from build123d import *

# Parameters (mm, degrees)
SKETCH_1_R      = 3.5
SKETCH_1_W      = 9.2
SKETCH_1_H      = 9.2
EXTRUDE_3_DEPTH = 100


with BuildPart() as part:
    # 草图1 → 凸台-拉伸3 (new body)
    with BuildSketch(Plane.XY):
        with BuildLine():
            Line((-27, 17), (-27, 9.314213562))
            Line((-27, 9.314213562), (-26.241421356, 9.314213562))
            ThreePointArc((-26.241421356, 9.314213562), (-26.149033403, 9.252481906), (-26.170710678, 9.143502884))
            Line((-26.170710678, 9.143502884), (-26.707106781, 8.607106781))
            Line((-26.707106781, 8.607106781), (-22.086856928, 3.986856928))
            ThreePointArc((-22.086856928, 3.986856928), (-20, 4.5), (-17.913143072, 3.986856928))
            Line((-17.913143072, 3.986856928), (-13.292893219, 8.607106781))
            Line((-13.292893219, 8.607106781), (-13.829289322, 9.143502884))
            ThreePointArc((-13.829289322, 9.143502884), (-13.850966597, 9.252481906), (-13.758578644, 9.314213562))
            Line((-13.758578644, 9.314213562), (-13, 9.314213562))
            Line((-13, 9.314213562), (-13, 17))
            Line((-13, 17), (-14.95, 17))
            Line((-14.95, 17), (-14.95, 18.5))
            ThreePointArc((-14.95, 18.5), (-14.510660172, 19.560660172), (-13.45, 20))
            Line((-13.45, 20), (13.45, 20))
            ThreePointArc((13.45, 20), (14.510660172, 19.560660172), (14.95, 18.5))
            Line((14.95, 18.5), (14.95, 17))
            Line((14.95, 17), (13, 17))
            Line((13, 17), (13, 9.314213562))
            Line((13, 9.314213562), (13.758578644, 9.314213562))
            ThreePointArc((13.758578644, 9.314213562), (13.850966597, 9.252481906), (13.829289322, 9.143502884))
            Line((13.829289322, 9.143502884), (13.292893219, 8.607106781))
            Line((13.292893219, 8.607106781), (17.913143072, 3.986856928))
            ThreePointArc((17.913143072, 3.986856928), (20, 4.5), (22.086856928, 3.986856928))
            Line((22.086856928, 3.986856928), (26.707106781, 8.607106781))
            Line((26.707106781, 8.607106781), (26.170710678, 9.143502884))
            ThreePointArc((26.170710678, 9.143502884), (26.149033403, 9.252481906), (26.241421356, 9.314213562))
            Line((26.241421356, 9.314213562), (27, 9.314213562))
            Line((27, 9.314213562), (27, 17))
            Line((27, 17), (25.05, 17))
            Line((25.05, 17), (25.05, 18.5))
            ThreePointArc((25.05, 18.5), (25.489339828, 19.560660172), (26.55, 20))
            Line((26.55, 20), (40, 20))
            Line((40, 20), (40, 6.55))
            ThreePointArc((40, 6.55), (39.560660172, 5.489339828), (38.5, 5.05))
            Line((38.5, 5.05), (37, 5.05))
            Line((37, 5.05), (37, 7))
            Line((37, 7), (29.314213562, 7))
            Line((29.314213562, 7), (29.314213562, 6.241421356))
            ThreePointArc((29.314213562, 6.241421356), (29.252481906, 6.149033403), (29.143502884, 6.170710678))
            Line((29.143502884, 6.170710678), (28.607106781, 6.707106781))
            Line((28.607106781, 6.707106781), (23.986856928, 2.086856928))
            ThreePointArc((23.986856928, 2.086856928), (24.5, 0), (23.986856928, -2.086856928))
            Line((23.986856928, -2.086856928), (28.607106781, -6.707106781))
            Line((28.607106781, -6.707106781), (29.143502884, -6.170710678))
            ThreePointArc((29.143502884, -6.170710678), (29.252481906, -6.149033403), (29.314213562, -6.241421356))
            Line((29.314213562, -6.241421356), (29.314213562, -7))
            Line((29.314213562, -7), (37, -7))
            Line((37, -7), (37, -5.05))
            Line((37, -5.05), (38.5, -5.05))
            ThreePointArc((38.5, -5.05), (39.560660172, -5.489339828), (40, -6.55))
            Line((40, -6.55), (40, -20))
            Line((40, -20), (26.55, -20))
            ThreePointArc((26.55, -20), (25.489339828, -19.560660172), (25.05, -18.5))
            Line((25.05, -18.5), (25.05, -17))
            Line((25.05, -17), (27, -17))
            Line((27, -17), (27, -9.314213562))
            Line((27, -9.314213562), (26.241421356, -9.314213562))
            ThreePointArc((26.241421356, -9.314213562), (26.149033403, -9.252481906), (26.170710678, -9.143502884))
            Line((26.170710678, -9.143502884), (26.707106781, -8.607106781))
            Line((26.707106781, -8.607106781), (22.086856928, -3.986856928))
            ThreePointArc((22.086856928, -3.986856928), (20, -4.5), (17.913143072, -3.986856928))
            Line((17.913143072, -3.986856928), (13.292893219, -8.607106781))
            Line((13.292893219, -8.607106781), (13.829289322, -9.143502884))
            ThreePointArc((13.829289322, -9.143502884), (13.850966597, -9.252481906), (13.758578644, -9.314213562))
            Line((13.758578644, -9.314213562), (13, -9.314213562))
            Line((13, -9.314213562), (13, -17))
            Line((13, -17), (14.95, -17))
            Line((14.95, -17), (14.95, -18.5))
            ThreePointArc((14.95, -18.5), (14.510660172, -19.560660172), (13.45, -20))
            Line((13.45, -20), (-13.45, -20))
            ThreePointArc((-13.45, -20), (-14.510660172, -19.560660172), (-14.95, -18.5))
            Line((-14.95, -18.5), (-14.95, -17))
            Line((-14.95, -17), (-13, -17))
            Line((-13, -17), (-13, -9.314213562))
            Line((-13, -9.314213562), (-13.758578644, -9.314213562))
            ThreePointArc((-13.758578644, -9.314213562), (-13.850966597, -9.252481906), (-13.829289322, -9.143502884))
            Line((-13.829289322, -9.143502884), (-13.292893219, -8.607106781))
            Line((-13.292893219, -8.607106781), (-17.913143072, -3.986856928))
            ThreePointArc((-17.913143072, -3.986856928), (-20, -4.5), (-22.086856928, -3.986856928))
            Line((-22.086856928, -3.986856928), (-26.707106781, -8.607106781))
            Line((-26.707106781, -8.607106781), (-26.170710678, -9.143502884))
            ThreePointArc((-26.170710678, -9.143502884), (-26.149033403, -9.252481906), (-26.241421356, -9.314213562))
            Line((-26.241421356, -9.314213562), (-27, -9.314213562))
            Line((-27, -9.314213562), (-27, -17))
            Line((-27, -17), (-25.05, -17))
            Line((-25.05, -17), (-25.05, -18.5))
            ThreePointArc((-25.05, -18.5), (-25.489339828, -19.560660172), (-26.55, -20))
            Line((-26.55, -20), (-40, -20))
            Line((-40, -20), (-40, -6.55))
            ThreePointArc((-40, -6.55), (-39.560660172, -5.489339828), (-38.5, -5.05))
            Line((-38.5, -5.05), (-37, -5.05))
            Line((-37, -5.05), (-37, -7))
            Line((-37, -7), (-29.314213562, -7))
            Line((-29.314213562, -7), (-29.314213562, -6.241421356))
            ThreePointArc((-29.314213562, -6.241421356), (-29.252481906, -6.149033403), (-29.143502884, -6.170710678))
            Line((-29.143502884, -6.170710678), (-28.607106781, -6.707106781))
            Line((-28.607106781, -6.707106781), (-23.986856928, -2.086856928))
            ThreePointArc((-23.986856928, -2.086856928), (-24.5, 0), (-23.986856928, 2.086856928))
            Line((-23.986856928, 2.086856928), (-28.607106781, 6.707106781))
            Line((-28.607106781, 6.707106781), (-29.143502884, 6.170710678))
            ThreePointArc((-29.143502884, 6.170710678), (-29.252481906, 6.149033403), (-29.314213562, 6.241421356))
            Line((-29.314213562, 6.241421356), (-29.314213562, 7))
            Line((-29.314213562, 7), (-37, 7))
            Line((-37, 7), (-37, 5.05))
            Line((-37, 5.05), (-38.5, 5.05))
            ThreePointArc((-38.5, 5.05), (-39.560660172, 5.489339828), (-40, 6.55))
            Line((-40, 6.55), (-40, 20))
            Line((-40, 20), (-26.55, 20))
            ThreePointArc((-26.55, 20), (-25.489339828, 19.560660172), (-25.05, 18.5))
            Line((-25.05, 18.5), (-25.05, 17))
            Line((-25.05, 17), (-27, 17))
        make_face()
        with Locations((-20, 0)):
            Circle(SKETCH_1_R, mode=Mode.SUBTRACT)
        with Locations(Location((20, 0, 0), (0, 0, 180))):
            Circle(SKETCH_1_R, mode=Mode.SUBTRACT)
        with Locations((-33.5, 13.5)):
            Rectangle(SKETCH_1_W, SKETCH_1_H, mode=Mode.SUBTRACT)
        with BuildLine():
            Line((-11.978679656, 6.121320344), (-16.013143072, 2.086856928))
            ThreePointArc((-16.013143072, 2.086856928), (-15.5, 0), (-16.013143072, -2.086856928))
            Line((-16.013143072, -2.086856928), (-11.978679656, -6.121320344))
            ThreePointArc((-11.978679656, -6.121320344), (-11.328361402, -7.09459039), (-11.1, -8.242640687))
            Line((-11.1, -8.242640687), (-11.1, -18.1))
            Line((-11.1, -18.1), (11.1, -18.1))
            Line((11.1, -18.1), (11.1, -8.242640687))
            ThreePointArc((11.1, -8.242640687), (11.328361402, -7.09459039), (11.978679656, -6.121320344))
            Line((11.978679656, -6.121320344), (16.013143072, -2.086856928))
            ThreePointArc((16.013143072, -2.086856928), (15.5, 0), (16.013143072, 2.086856928))
            Line((16.013143072, 2.086856928), (11.978679656, 6.121320344))
            ThreePointArc((11.978679656, 6.121320344), (11.328361402, 7.09459039), (11.1, 8.242640687))
            Line((11.1, 8.242640687), (11.1, 18.1))
            Line((11.1, 18.1), (-11.1, 18.1))
            Line((-11.1, 18.1), (-11.1, 8.242640687))
            ThreePointArc((-11.1, 8.242640687), (-11.328361402, 7.09459039), (-11.978679656, 6.121320344))
        make_face(mode=Mode.SUBTRACT)
        with Locations((-33.5, -13.5)):
            Rectangle(SKETCH_1_W, SKETCH_1_H, mode=Mode.SUBTRACT)
        with Locations((33.5, -13.5)):
            Rectangle(SKETCH_1_W, SKETCH_1_H, mode=Mode.SUBTRACT)
        with Locations((33.5, 13.5)):
            Rectangle(SKETCH_1_W, SKETCH_1_H, mode=Mode.SUBTRACT)
    extrude(amount=-EXTRUDE_3_DEPTH)


solid = part.part
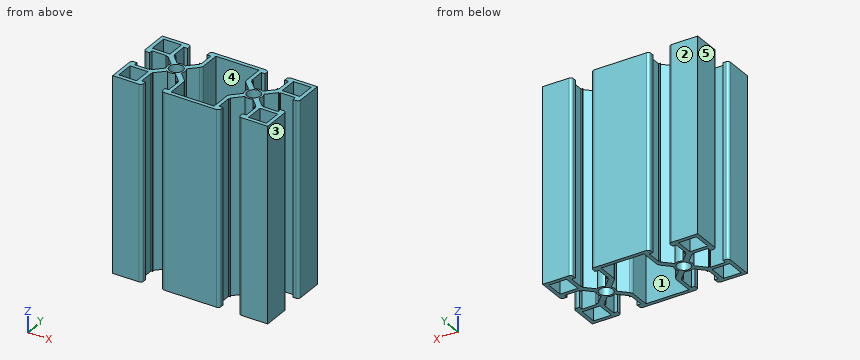
Input: part model. Units: mm. Frame: model coordinates. Face numbers are marked on the shaded views. A direction names the side the tool comes from. Give positions to 0.01 mm unless a question says otherwise; leave off trailing zeros. Loops run counter-clockwise (first coordinate to the right, second up) from the corner with the lowest first, then second, coordinate; pieces in that order, holes last. Notation, with made-up numbers: (2.5, 82) -> (32.5, 82) arc R24 cw to (32.5, 106) -> close; hole circle Ø11 at (51.5, 0). An arc over 180 degrees is marked (long way). Answer as a JSON object with one key per item and string values. Group by question number.
Item 1: Line query: probe 1 along X at (y, z) = (17.5, -75.5); probe 2 along X at (y, z) = (-12.5, -35.5); probe 3 along Y at (x, z) = (-34, -57.5). Output: solid intervals per line, ascending.
Item 2: Cut plane D-D, the plane x = -20. Return the cut outline in (y, z), and give its area (3 significant figures).
Item 3: Pull-direction query (X, two-part tool) for the marked faces 1, 2 and 3; classes: released by +X, released by -X, zero draft, split by the parting line, or undercut.
Item 4: Cut plane B-B, the plane x = -1.5. Return the cut outline in (y, z), and give its area (3 significant figures).
Item 5: Reachability of the marked faces 4 and 5 from +Z, -Z, +X, -X, +Y, -Y: full face, straight path, thin tool, end or side. Return the list, or none.
Item 6: Cut plane A-A, the plane y = 0. Return the cut outline in (x, z), and give its area (3 significant figures).
Item 7: Cut plane C-C, the plane x = 31. Return the cut outline in (y, z).
Item 8: Pin query (flat end, axial travel): P1, Ø3, axis at y = 0.5, z = -18, coming from the +X side; P2, Ø1, axis at y = 5.5, z = -30.5, coming from the +X side. Return the tip coordinate at first contact, or that it passes through.
Checks:
{
 "1": {"probe 1": "x = -40 to -38.1, -28.9 to -25.05, -14.95 to -11.1, 11.1 to 14.95, 25.05 to 28.9, 38.1 to 40", "probe 2": "x = -40 to -38.1, -28.9 to -27, -13 to -11.1, 11.1 to 13, 27 to 28.9, 38.1 to 40", "probe 3": "y = -20 to -18.1, -8.9 to -7, 7 to 8.9, 18.1 to 20"},
 "2": {"outline": "(-4.5, -100) -> (-3.5, -100) -> (-3.5, 0) -> (-4.5, 0) -> close; (3.5, -100) -> (4.5, -100) -> (4.5, 0) -> (3.5, 0) -> close", "area": "200 mm²"},
 "3": {"face 1": "undercut", "face 2": "zero draft", "face 3": "released by +X"},
 "4": {"outline": "(-20, -100) -> (-18.1, -100) -> (-18.1, 0) -> (-20, 0) -> close; (18.1, -100) -> (20, -100) -> (20, 0) -> (18.1, 0) -> close", "area": "380 mm²"},
 "5": {"face 4": "+Z, -Z", "face 5": "+Z, -Z, -X, +Y, -Y"},
 "6": {"outline": "(-24.5, -100) -> (-23.5, -100) -> (-23.5, 0) -> (-24.5, 0) -> close; (-16.5, -100) -> (-15.5, -100) -> (-15.5, 0) -> (-16.5, 0) -> close; (15.5, -100) -> (16.5, -100) -> (16.5, 0) -> (15.5, 0) -> close; (23.5, -100) -> (24.5, -100) -> (24.5, 0) -> (23.5, 0) -> close", "area": "400 mm²"},
 "7": {"outline": "(-20, -100) -> (-18.1, -100) -> (-18.1, 0) -> (-20, 0) -> close; (-8.9, -100) -> (-7, -100) -> (-7, 0) -> (-8.9, 0) -> close; (7, -100) -> (8.9, -100) -> (8.9, 0) -> (7, 0) -> close; (18.1, -100) -> (20, -100) -> (20, 0) -> (18.1, 0) -> close"},
 "8": {"P1": "stops at x = 24.5", "P2": "stops at x = 39.9"}
}
